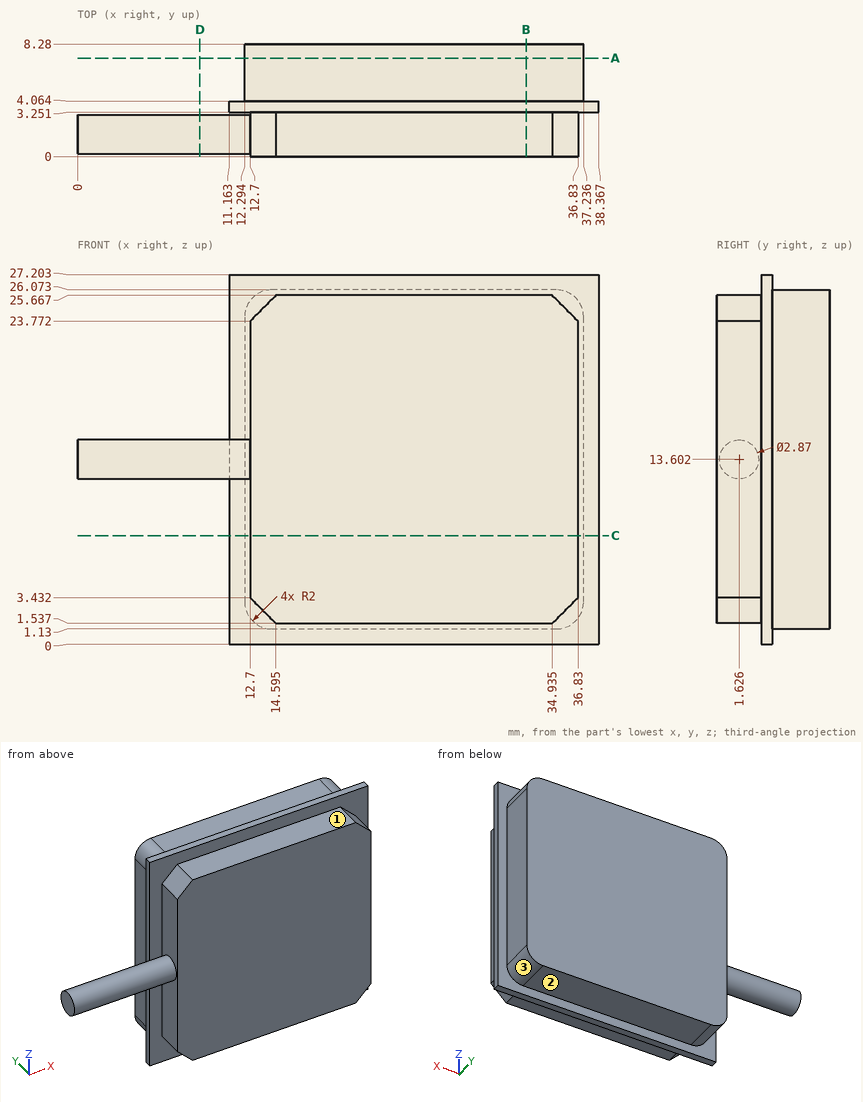
The figure shows three views and two pictorial views of one solid part (mm, origin at its lowest corner). Answer the questions. A direction names the side the tool comes from. Round coordinates to 2 decimals unless told otherwise and drop trailing zeros. Write each loop counter-clockwise with the first axis right and the second up, starting at its lowest first coordinate (ties: lowest second). Pieces come first, ordered by that corner, then holes. Notation, with made-up numbers: (-34, 14) -> (6, 14) arc R18 cw to (6, 20) -> close; hole circle Ø9 at (-22.5, 89). An arc over 180 degrees is marked (long way). Answer as a JSON object with one key per item and string values. Group by question number.
Q1. Which of the six approach directions +Z, -Z, +X, -X, +Y, -Y give full straight-line access (tool end or side, diameter ignored) to the marked faces 1, 2 and 3?
Q2. Straight lines are drawn through the part: line 1 along Z through (x, y) = (15, 7.75); line 2 along Y through (x, z) = (12.5, 19.5); line 3 along X through (y, z) = (5, 10.5). For each, find the intervals that lie inside material, in ascending order.
Q3. Section C-C (z = 8) is taken. Write down the section's boundary in (x, y), plus the area to 3 significant figures.
Q4. Section A-A (y = 7.25) is taken. Write down the section's boundary in (x, z).
Q5. Section B-B (x = 33) is taken. Write down the section's boundary in (y, z).
Q6. Each of these flat-tipped pins is pushed along its axis until it touches: pin 1 Ø1 at (x, y) = (21, 1.5) entering from +Z; pin 2 Ø1.3 at (y, z) = (7, 15) entering from +X; pin 3 Ø2 at (y, z) = (6, 13.5) entering from -X. Where does it stop, or does it pass through?
Q7. Section D-D (x = 9) is taken. Write down the section's boundary in (y, z) (1 decimal).
Check values:
{
 "1": {"face 1": "+Z, +X, -X, -Y", "face 2": "-Z, +X, -X, +Y", "face 3": "-Z, +X, +Y"},
 "2": {"line 1": "1.13 to 26.07", "line 2": "3.25 to 8.28", "line 3": "12.29 to 37.24"},
 "3": {"outline": "(11.16, 3.25) -> (12.7, 3.25) -> (12.7, 0) -> (36.83, 0) -> (36.83, 3.25) -> (38.37, 3.25) -> (38.37, 4.06) -> (37.24, 4.06) -> (37.24, 8.28) -> (12.29, 8.28) -> (12.29, 4.06) -> (11.16, 4.06) -> close", "area": "206 mm^2"},
 "4": {"outline": "(12.29, 3.13) arc R2 ccw to (14.29, 1.13) -> (35.24, 1.13) arc R2 ccw to (37.24, 3.13) -> (37.24, 24.07) arc R2 ccw to (35.24, 26.07) -> (14.29, 26.07) arc R2 ccw to (12.29, 24.07) -> close"},
 "5": {"outline": "(0, 1.54) -> (3.25, 1.54) -> (3.25, 0) -> (4.06, 0) -> (4.06, 1.13) -> (8.28, 1.13) -> (8.28, 26.07) -> (4.06, 26.07) -> (4.06, 27.2) -> (3.25, 27.2) -> (3.25, 25.67) -> (0, 25.67) -> close"},
 "6": {"pin 1": "z = 25.67", "pin 2": "x = 37.24", "pin 3": "x = 12.29"},
 "7": {"outline": "circle Ø2.9 at (1.6, 13.6)"}
}
